Could you check a few things on this model? Use its own coordinates, in mm. Face numbers are marked on the shaded views. A direction names the side the tool comes from. Give positions to 0.01 mm unless a question says otherwise; leave off trailing zeros. Order: outer loops, then holes, each group sorted by start corner. A loop starts at its lowest first (then second) coordinate and runs counter-clockwise, first axis right, second up.
(1) On a 3-axis mill with a long thin cutter (end or side, diameter ignored), from which of +Z, -Z, +X, -X, +Y, -Y can I reach the whole of each face in a straight line? I mean the marked faces 4, 5, 6, 7 and 8. Say none if no direction works.
(2) Imagine slicing it at A-A, the plane x = 0. State how many separate pieces and enclosed holes the cut face has, then the cut area to 3 significant figures.
(3) If we mould it in two halves opening along Y, with no side actions, what happens to the marked faces 1, 2 and 3? For each: released by +Y, released by -Y, zero draft, split by the parting line, or undercut.
(4) Will these pins go through, and if not, where does the flat tip stop? pin 1 (0.8 mm diameter, centred on x = 0.5, y = 1.5, fed in from -Z); pin 2 (2 mm diameter, centred on x = 10.5, z = 1.5, fed in from -Y); pin 3 (0.8 mm diameter, centred on y = 2, z = -10, fed in from +X).
(5) If I drill on probe 1 along Y at (x, z) = (-1.5, -6); probe 2 along X at (y, z) = (1.6, 0); probe 3 along Z at (x, y) = (2.5, -0.75), over which ranges is the centre line in solid material (lowest first)?
(6) Imagine slicing it at C-C, the plane y = -1.5. Write out the boundary of the cut face in (x, z).
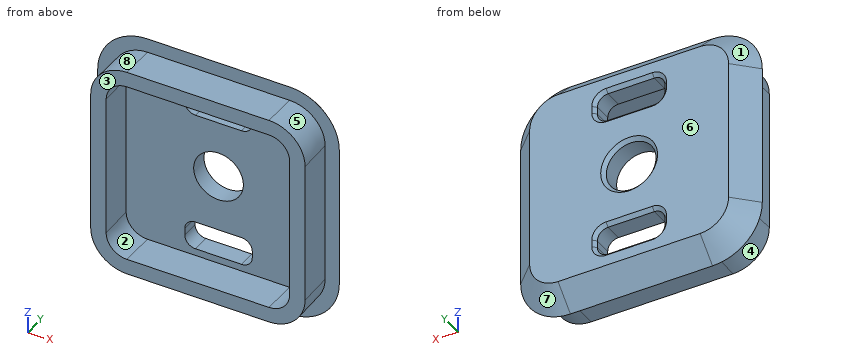
from build123d import *

# Parameters (mm, degrees)
CROQUIS1_W                 = 34
CROQUIS1_H                 = 34
SALIENTE_EXTRUIR1_DEPTH    = 3
REDONDEO1_R                = 7
CHAFL_N1_SIZE              = 3
CROQUIS2_W                 = 9.5
CROQUIS2_H                 = 4
CORTAR_EXTRUIR1_DEPTH      = 25.228082879
REDONDEO2_R                = 1.5
CHAFL_N2_SIZE              = 0.5
SALIENTE_EXTRUIR2_DEPTH    = 5
SALIENTE_EXTRUIR2_DRAFT    = -1
CROQUIS9_R                 = 3.5
CORTAR_EXTRUIR2_DEPTH      = 26.337718919
CHAFL_N3_SIZE              = 0.5
REDONDEO2_OF_SIMETR_A1_R   = 1.5
CHAFL_N2_OF_SIMETR_A1_SIZE = 0.5


with BuildPart() as part:
    # Croquis1 → Saliente-Extruir1 (new body)
    with BuildSketch(Plane(origin=(0, 0, 0), x_dir=(1, 0, 0), z_dir=(0, 1, 0))):
        Rectangle(CROQUIS1_W, CROQUIS1_H)
    extrude(amount=SALIENTE_EXTRUIR1_DEPTH)

    # Redondeo1
    redondeo1_edges = [part.edges().sort_by_distance(p)[0] for p in [
        (17, 1.5, 17),
        (-17, 1.5, 17),
        (-17, 1.5, -17),
        (17, 1.5, -17),
    ]]
    fillet(redondeo1_edges, radius=REDONDEO1_R)

    # Chaflán1
    chafl_n1_edges = [part.edges().sort_by_distance(p)[0] for p in [
        (17, 3, 0),
        (14.949747468, 3, -14.949747468),
        (14.949747468, 3, 14.949747468),
        (0, 3, -17),
        (0, 3, 17),
        (-14.949747468, 3, -14.949747468),
        (-14.949747468, 3, 14.949747468),
        (-17, 3, 0),
    ]]
    chamfer(chafl_n1_edges, length=CHAFL_N1_SIZE - 0.0001)  # a hair under: the kernel refuses the full size

    # Croquis2 → Cortar-Extruir1 (cut, through all)
    with BuildSketch(Plane(origin=(0, 3, 0), x_dir=(1, 0, 0), z_dir=(0, 1, 0))):
        with Locations((0, 10)):
            Rectangle(CROQUIS2_W, CROQUIS2_H)
    cortar_extruir1 = extrude(amount=-CORTAR_EXTRUIR1_DEPTH, mode=Mode.SUBTRACT)

    # Redondeo2
    redondeo2_edges = [part.edges().sort_by_distance(p)[0] for p in [
        (4.75, 1.5, -12),
        (4.75, 1.5, -8),
        (-4.75, 1.5, -8),
        (-4.75, 1.5, -12),
    ]]
    fillet(redondeo2_edges, radius=REDONDEO2_R)

    # Chaflán2
    chafl_n2_edges = [part.edges().sort_by_distance(p)[0] for p in [
        (0, 3, -8),
        (-4.75, 3, -10),
        (4.75, 3, -10),
        (0, 3, -12),
        (-4.310660172, 3, -8.439339828),
        (4.310660172, 3, -8.439339828),
        (4.310660172, 3, -11.560660172),
        (-4.310660172, 3, -11.560660172),
    ]]
    chamfer(chafl_n2_edges, length=CHAFL_N2_SIZE)


with BuildPart() as saliente_extruir2_tool:
    # Croquis8 → Saliente-Extruir2 (with draft: the straight prism first)
    with BuildSketch(Plane.XZ):
        with BuildLine():
            ThreePointArc((-10, 15), (-13.535533906, 13.535533906), (-15, 10))
            Line((-15, 10), (-15, -10))
            ThreePointArc((-15, -10), (-13.535533906, -13.535533906), (-10, -15))
            Line((-10, -15), (10, -15))
            ThreePointArc((10, -15), (13.535533906, -13.535533906), (15, -10))
            Line((15, -10), (15, 10))
            ThreePointArc((15, 10), (13.535533906, 13.535533906), (10, 15))
            Line((10, 15), (-10, 15))
        make_face()
        with BuildLine():
            Line((-13, 10), (-13, -10))
            ThreePointArc((-13, -10), (-12.121320344, -12.121320344), (-10, -13))
            Line((-10, -13), (10, -13))
            ThreePointArc((10, -13), (12.121320344, -12.121320344), (13, -10))
            Line((13, -10), (13, 10))
            ThreePointArc((13, 10), (12.121320344, 12.121320344), (10, 13))
            Line((10, 13), (-10, 13))
            ThreePointArc((-10, 13), (-12.121320344, 12.121320344), (-13, 10))
        make_face(mode=Mode.SUBTRACT)
    extrude(amount=SALIENTE_EXTRUIR2_DEPTH)
    # Saliente-Extruir2: the draft: its side faces are tilted about the plane it starts from
    saliente_extruir2_sides = [saliente_extruir2_tool.faces().sort_by_distance(p)[0] for p in [
        (0, -2.5, 15),
        (-13.535533906, -2.5, 13.535533906),
        (-15, -2.5, 0),
        (-13.535533906, -2.5, -13.535533906),
        (0, -2.5, -15),
        (13.535533906, -2.5, -13.535533906),
        (15, -2.5, 0),
        (13.535533906, -2.5, 13.535533906),
        (12.121320344, -2.5, 12.121320344),
        (13, -2.5, 0),
        (12.121320344, -2.5, -12.121320344),
        (0, -2.5, -13),
        (-12.121320344, -2.5, -12.121320344),
        (-13, -2.5, 0),
        (-12.121320344, -2.5, 12.121320344),
        (0, -2.5, 13),
    ]]
    draft(saliente_extruir2_sides, Plane.XZ, SALIENTE_EXTRUIR2_DRAFT)


with BuildPart() as part_1:
    add(part.part)

    # Saliente-Extruir2: add saliente_extruir2_tool
    add(saliente_extruir2_tool.part)

    # Croquis9 → Cortar-Extruir2 (cut, through all)
    with BuildSketch(Plane(origin=(0, 3, 0), x_dir=(1, 0, 0), z_dir=(0, 1, 0))):
        with Locations(Location((0, 0, 0), (0, 0, 270))):
            Circle(CROQUIS9_R)
    extrude(amount=-CORTAR_EXTRUIR2_DEPTH, mode=Mode.SUBTRACT)

    # Chaflán3
    chafl_n3_edges = [part_1.edges().sort_by_distance(p)[0] for p in [
        (0, 3, -3.5),
    ]]
    chamfer(chafl_n3_edges, length=CHAFL_N3_SIZE)

    # Simetría1: Cortar-Extruir1 across plane
    add(cortar_extruir1.mirror(Plane.XY), mode=Mode.SUBTRACT)

    # Redondeo2 of Simetría1
    redondeo2_of_simetr_a1_edges = [part_1.edges().sort_by_distance(p)[0] for p in [
        (4.75, 1.5, 12),
        (4.75, 1.5, 8),
        (-4.75, 1.5, 8),
        (-4.75, 1.5, 12),
    ]]
    fillet(redondeo2_of_simetr_a1_edges, radius=REDONDEO2_OF_SIMETR_A1_R)

    # Chaflán2 of Simetría1
    chafl_n2_of_simetr_a1_edges = [part_1.edges().sort_by_distance(p)[0] for p in [
        (0, 3, 8),
        (-4.75, 3, 10),
        (4.75, 3, 10),
        (0, 3, 12),
        (-4.310660172, 3, 8.439339828),
        (4.310660172, 3, 8.439339828),
        (4.310660172, 3, 11.560660172),
        (-4.310660172, 3, 11.560660172),
    ]]
    chamfer(chafl_n2_of_simetr_a1_edges, length=CHAFL_N2_OF_SIMETR_A1_SIZE)


solid = part_1.part
Answer block:
1. face 4: -Z, -X
1. face 5: +Z, +X
1. face 6: +Z, -Z, +X, -X, +Y
1. face 7: -Z, +X, +Y
1. face 8: +Z, -X
2. separate pieces: 4
2. enclosed holes: 0
2. area: 68.1 mm2
3. face 1: released by +Y
3. face 2: undercut
3. face 3: released by -Y
4. pin 1: stops at z = -15.9
4. pin 2: stops at y = 0
4. pin 3: stops at x = 15.4
5. probe 1: y = 0 to 3
5. probe 2: x = -15.4 to -3.5, 3.5 to 15.4
5. probe 3: z = -15.01 to -12.99, 12.99 to 15.01
6. outline: (-15.03, -10) arc R5.03 ccw to (-10, -15.03) - (10, -15.03) arc R5.03 ccw to (15.03, -10) - (15.03, 10) arc R5.03 ccw to (10, 15.03) - (-10, 15.03) arc R5.03 ccw to (-15.03, 10) - close; hole (-12.97, -10) arc R2.97 ccw to (-10, -12.97) - (10, -12.97) arc R2.97 ccw to (12.97, -10) - (12.97, 10) arc R2.97 ccw to (10, 12.97) - (-10, 12.97) arc R2.97 ccw to (-12.97, 10) - close
